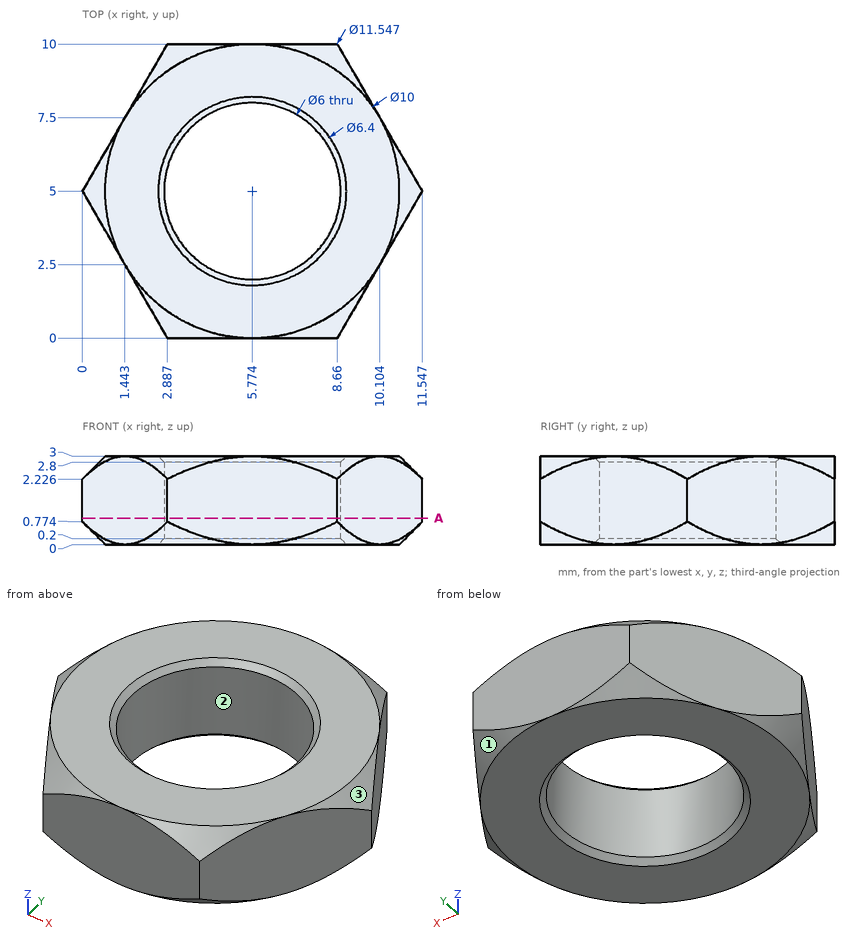
Source: three-view drawing plus pictorial views. Frame: mm from the lowest corner of the part. Round coordinates to 2 decimals unless told otherwise and drop trailing zeros. Order: outer loops, then holes, each group sorted by start corner. A loop starts at its lowest first (then second) coordinate and runs counter-clockwise, first axis right, second up. Notation, with made-up numbers: (68, 80.25) - (92, 80.25) arc R26 cw to (92, 103.25) - close; hole circle Ø4 at (70.5, -10.5). An arc over 180 degrees is marked (long way). Answer in a Markdown table with one row per item.
Item 1: Section query A-A (z = 0.9). Return the cut outline in (x, y).
Model answer:
| item | result |
|---|---|
| outline | (0, 5) - (2.89, 0) - (8.66, 0) - (11.55, 5) - (8.66, 10) - (2.89, 10) - close; hole circle Ø6 at (5.77, 5) |
Item 2: Mould query, pull axis Y, two halves, no side actions, for the marked faces 1, 2 and 3. Classes: released by +Y, released by -Y, zero draft, split by the parting line, or undercut.
Model answer:
| item | result |
|---|---|
| face 1 | released by +Y |
| face 2 | undercut |
| face 3 | split by the parting line |
Item 3: Line query: line 1 (Y direction, x = 7.5, z = 2.4) (1 decimal); line 2 (X direction, y = 7.75, z = 2.55) (1 decimal); line 3 (X direction, y = 5.75, z = 0.95) (1 decimal). Output: solid intervals per line, ascending.
Model answer:
| item | result |
|---|---|
| line 1 | y = 0 to 2.5, 7.5 to 10 |
| line 2 | x = 1.6 to 4.6, 7 to 10 |
| line 3 | x = 0.4 to 2.9, 8.7 to 11.1 |
